Autodesk Inventor part; units mm, degrees
ref_plane "YZ Plane" through (0, 0, 0) normal (1, 0, 0) x (0, 1, 0)
ref_plane "XZ Plane" through (0, 0, 0) normal (0, 1, 0) x (-1, 0, 0)
ref_plane "XY Plane" through (0, 0, 0) normal (0, 0, 1) x (1, 0, 0)
sketch "Sketch1" plane through (0, 0, 0) normal (0, 1, 0) x (-1, 0, 0)
  circle A0 centre (0, 0) radius 2.6
  circle A1 centre (0, 0) radius 4
  circle A2 centre (0, 0) radius 15
  circle A3 centre (0, 0) radius 13
  dimension "d21" = 5.2
  dimension "d22" = 8
  dimension "d23" = 30
  dimension "d31" = 2
extrude "Extrusion6" add sketch "Sketch1" against normal blind 1.5 contours A1 | A2 | A3
extrude "Extrusion7" add sketch "Sketch1" along normal blind 0.45 contours A1
chamfer "Chamfer1" distance 0.25 angle 60 1 edges at (4, 0, 0) measured on face at (-11.188, 0, -1.1966)
extrude "Extrusion8" add sketch "Sketch1" along normal blind 0.3 contours A2
properties part number "071_0204_RollCutter20mmScrewClamp8mm"
Can you work these out from the model? Positions are in its coordinate system, mm. Give positions to 0.01 mm unless a question says otherwise; leave off trailing zeros. Loops run counter-clockwise (first coordinate to the right, second up) from the corner with the lowest first, then second, coordinate; pieces in that order, holes last. Notation, with made-up numbers: M -4,-13.75 L 2,-13.75 A26 cw 2,20.25 Z; hole C 83.5,85.25 d11. An arc over 180 degrees is marked long. Answer in a Markdown table with one row per item.
1. Suppose I cut it at D-D on y = -0.4. Write out the boundary of the cut face in (x, z), plus the area to 3 significant figures.
Taken from the geometry:
| item | result |
|---|---|
| outline | C 0,0 d30; hole C 0,0 d5.2 |
| area | 686 mm² |
2. Thinking about a two-plate mould opening in X: for faces 1 (the flat face through (0, -1.5, -3)), 2 (the flat face through (-6, 0, 0)), 3 (the cylindrical face through (14.985, -0.587, 0.66)), which applies, released by +X, released by -X, zero draft, split by the parting line, or undercut?
Taken from the geometry:
| item | result |
|---|---|
| face 1 | zero draft |
| face 2 | undercut |
| face 3 | split by the parting line |
3. For pin 1 Ø1 at (y, z) = (0, -6) entering from +X, with a flat end and sliding along its axis, tell me the tip position at first contact or that it passes through.
Taken from the geometry:
| item | result |
|---|---|
| pin 1 | stops at x = 13.96 |
4. If I drill on line 1 along Z through (x, y) = (0, -0.8); line 2 along Y through (x, z) = (-1.75, 10.75); line 3 along Y through (x, z) = (13.75, 5.75), over which ranges is the centre line in solid material (lowest first)?
Taken from the geometry:
| item | result |
|---|---|
| line 1 | z = -15 to -2.6, 2.6 to 15 |
| line 2 | y = -1.5 to 0 |
| line 3 | y = -1.5 to 0.3 |
5. Suppose I cut it at C-C on z = -12. Write out the boundary of the cut face in (x, y).
Taken from the geometry:
| item | result |
|---|---|
| outline | M -9,-1.5 L 9,-1.5 L 9,0.3 L 5,0.3 L 5,0 L -5,0 L -5,0.3 L -9,0.3 Z |
